```python
from build123d import *

# Parameters (mm, degrees)
SKETCH1_W           = 508
SKETCH1_H           = 127
BOSS_EXTRUDE1_DEPTH = 76.2
SKETCH5_W           = 120.904
SKETCH5_H           = 70.104
CUT_EXTRUDE1_DEPTH  = 509
FILLET1_R           = 3.81
SKETCH9_R           = 15.875
CUT_EXTRUDE5_DEPTH  = 128


with BuildPart() as part:
    # Sketch1 → Boss-Extrude1 (new body)
    with BuildSketch(Plane(origin=(0, 0, 0), x_dir=(1, 0, 0), z_dir=(0, 1, 0))):
        with Locations((-33.748251748, 0.444055944)):
            Rectangle(SKETCH1_W, SKETCH1_H)
    extrude(amount=BOSS_EXTRUDE1_DEPTH)

    # Sketch5 → Cut-Extrude1 (cut, through all)
    with BuildSketch(Plane.ZY.offset(287.748251748)):
        with Locations((-0.444055944, 38.1)):
            Rectangle(SKETCH5_W, SKETCH5_H)
    extrude(amount=-CUT_EXTRUDE1_DEPTH, mode=Mode.SUBTRACT)

    # Fillet1
    fillet1_edges = [part.edges().sort_by_distance(p)[0] for p in [
        (-33.748251748, 76.2, -63.944055944),
        (-33.748251748, 3.048, -60.896055944),
        (-33.748251748, 73.152, -60.896055944),
        (-33.748251748, 73.152, 60.007944056),
        (-33.748251748, 3.048, 60.007944056),
        (-33.748251748, 0, -63.944055944),
        (-33.748251748, 0, 63.055944056),
        (-33.748251748, 76.2, 63.055944056),
    ]]
    fillet(fillet1_edges, radius=FILLET1_R)

    # Sketch9 → Cut-Extrude5 (cut, through all)
    with BuildSketch(Plane.XY.offset(63.055944056)):
        with Locations((-224.248251748, 38.1)):
            Circle(SKETCH9_R)
    extrude(amount=-CUT_EXTRUDE5_DEPTH, mode=Mode.SUBTRACT)


solid = part.part
```
Can you work these out from the model? Positions are in its coordinate system, mm. A direction names the side the tool comes from. Coordinates: 2 decimals unless noted, no trailing zeros. Order: outer loops, then holes, each group sorted by start corner. A loop starts at its lowest first (then second) coordinate and runs counter-clockwise, first axis right, second up.
1. If we section it at C-C (y = 58.5): Please give me the cut outline in (x, z).
2. I need wall thicknesses on line 1 (Y direction, x = -31.5, z = -40); line 2 (Z direction, x = -264.5, y = 18.5); line 3 (X direction, y = 38, z = 61). Which ranges of each line are inside material? Lowest first, please.
3. If we section it at A-A (y = 38.1): Please give me the cut outline in (x, z), then the cut area to 3 significant figures.
4. If we section it at B-B (z = 26): Please give me the cut outline in (x, y), then the cut area to 3 significant figures.
5. If we section it at D-D (x = 60.5): Please give me the cut outline in (y, z).
6. For faces 1 (the face through (-37, 0, -1)), 2 (the face through (-37, 73.152, -1)), which set-ups out of +Z, -Z, +X, -X, +Y, -Y let a thin tool reach every point of the face, with its end or its side?
7. Thinking about a two-plate mould opening in Z: for faces 3 (the face through (-287.748, 75, 5)), 4 (the face through (-37, 38, -63.944)), 5 (the face through (-37, 3.048, -1)), which applies, +Z half, -Z half, draft (parallel to the pull), parting line (faces both ways), or undercut?
Entries:
1. outline: (-287.75, -63.94) - (220.25, -63.94) - (220.25, -60.9) - (-287.75, -60.9) - close; (-287.75, 60.01) - (220.25, 60.01) - (220.25, 63.06) - (-287.75, 63.06) - close
2. line 1: y = 0 to 3.05, 73.15 to 76.2
2. line 2: z = -63.94 to -60.9, 60.01 to 63.06
2. line 3: x = -287.75 to -240.12, -208.37 to 220.25
3. outline: (-287.75, -63.94) - (-240.12, -63.94) - (-240.12, -60.9) - (-287.75, -60.9) - close; (-287.75, 60.01) - (-240.12, 60.01) - (-240.12, 63.06) - (-287.75, 63.06) - close; (-208.37, -63.94) - (220.25, -63.94) - (220.25, -60.9) - (-208.37, -60.9) - close; (-208.37, 60.01) - (220.25, 60.01) - (220.25, 63.06) - (-208.37, 63.06) - close
3. area: 2,900 mm2
4. outline: (-287.75, 0) - (220.25, 0) - (220.25, 3.05) - (-287.75, 3.05) - close; (-287.75, 73.15) - (220.25, 73.15) - (220.25, 76.2) - (-287.75, 76.2) - close
4. area: 3,100 mm2
5. outline: (0, -60.13) arc R3.81 ccw to (3.81, -63.94) - (72.39, -63.94) arc R3.81 ccw to (76.2, -60.13) - (76.2, 59.25) arc R3.81 ccw to (72.39, 63.06) - (3.81, 63.06) arc R3.81 ccw to (0, 59.25) - close; hole (3.05, -57.09) arc R3.81 ccw to (6.86, -60.9) - (69.34, -60.9) arc R3.81 ccw to (73.15, -57.09) - (73.15, 56.2) arc R3.81 ccw to (69.34, 60.01) - (6.86, 60.01) arc R3.81 ccw to (3.05, 56.2) - close
6. face 1: +Z, -Z, +X, -X, -Y
6. face 2: +X, -X
7. face 3: draft
7. face 4: -Z half
7. face 5: undercut
